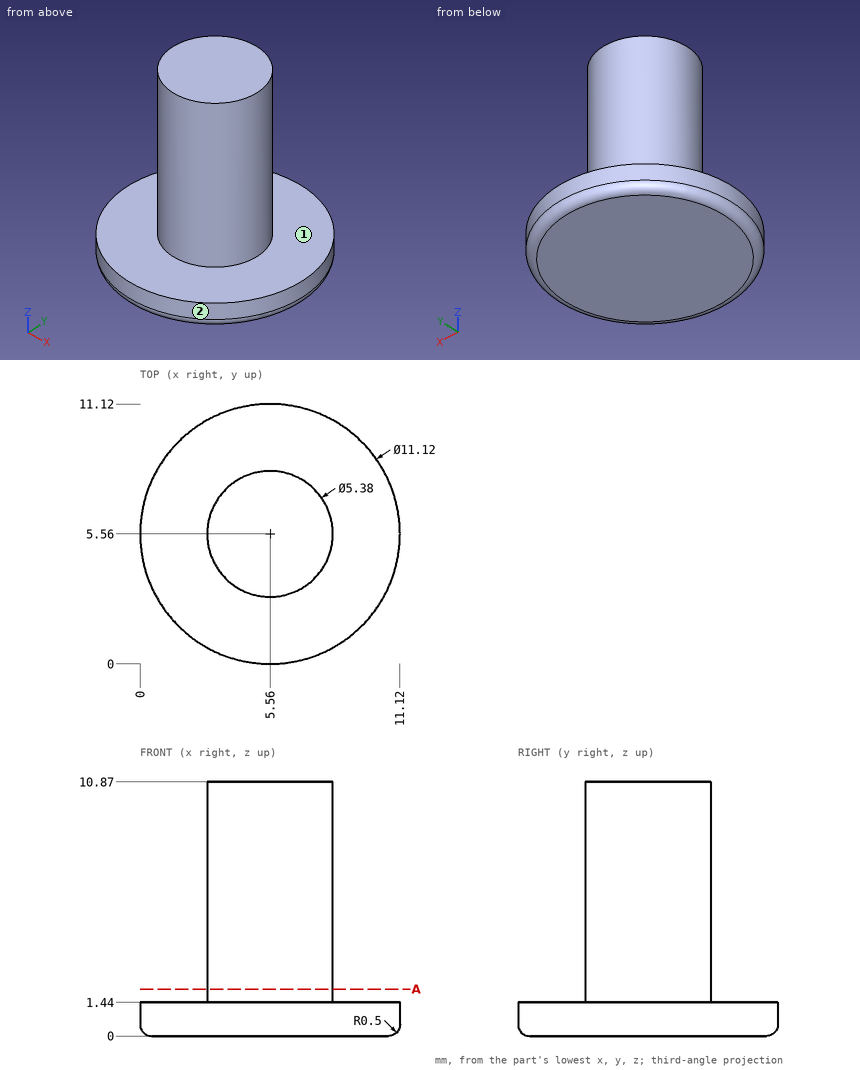
Job drawing, mm, ordinate dimensions from the low corner. One solid piece. A direction names the side the tool comes from. Round coordinates to 2 decimals unless told otherwise and drop trailing zeros. Loops run counter-clockwise (first coordinate to the right, second up) from the corner with the lowest first, then second, coordinate; pieces in that order, holes last. Notation, with made-up numbers: M 41.25,2 L 94.25,2 A30 cw 94.25,30 Z; hole C -18.75,57 d1. An arc over 180 degrees is marked long. One line per question, with ' | ' between items. Start each with the question number.
Item 1: Cut at A-A, the plane z = 2. Write the cut outline in (x, y).
Item 2: Wall check: line 1 (Z direction, x = 7, y = 3.25); line 2 (X direction, y = 5.5, z = 4.5); line 3 (Y direction, x = 3.25, z = 3.5). Give the ranges that are in metal, low to high.
Item 3: Which spindle directions (+Z, -Z, +X, -X, +Y, -Y) get a long thin tool onto all of the face, cutting with end or side? Do the marked faces 1 and 2. Say none if no direction does.
Item 4: Pin check, flat tips, straight feed: pin 1 Ø2 at (y, z) = (9.5, 5) entering from +X; pin 2 Ø1 at (y, z) = (5.5, 4) entering from -X; pin 3 Ø6 at (y, z) = (9.5, 5) entering from -X; pin 4 Ø6 at (y, z) = (2.5, 7.5) entering from +X. Stop position of each tip, or through.
Responses:
1) outline: C 5.56,5.56 d5.38
2) line 1: z = 0 to 1.44 | line 2: x = 2.87 to 8.25 | line 3: y = 4.18 to 6.94
3) face 1: +Z | face 2: +Z, -Z
4) pin 1: passes through | pin 2: stops at x = 2.87 | pin 3: stops at x = 3.04 | pin 4: stops at x = 8.25
